Drawing for the job (mm, zero at the part's lowest x, y, z). Round coordinates to 2 decimals unless told otherwise and drop trailing zeros. Loops run counter-clockwise (first coordinate to the right, second up) from the corner with the lowest first, then second, coordinate; pieces in that order, holes last. Notation, with made-up numbers: M 20,28.25 L 64,28.25 A26 cw 64,49.25 Z; hole C -17,57 d10. An arc over 180 degrees is marked long. Use a Markdown table: item, result. Add a question column.
Q1. Cut at C-C (z = 30). Give the cut face in (x, y), plus the area to 3 significant figures.
Q2. Cut at A-A (y = 15). Give the cut face in (x, z).
Q3. Probe line 1 (Y direction, x = 15, z = 29.5); line 2 (X direction, y = 18.5, z = 28.5); line 3 (Y direction, x = 16.5, z = 3.5). List the from-to ranges inside material, lowest first. Write a range as from..to.
Q4. Mould opens along X. For the marked faces 1, 2 and 3 say: +X half, -X half, draft (parallel to the pull), parting line (faces both ways), or undercut.
Q5. Pin check, flat tips, straight feed: pin 1 (1 mm diameter, centred on y = 6.5, z = 31.5, fed in from +X); pin 2 (6 mm diameter, centred on y = 11, z = 16.5, fed in from +X); pin 3 (5 mm diameter, centred on y = 23, z = 31.5, fed in from +X). Stop position of each tip, or through.
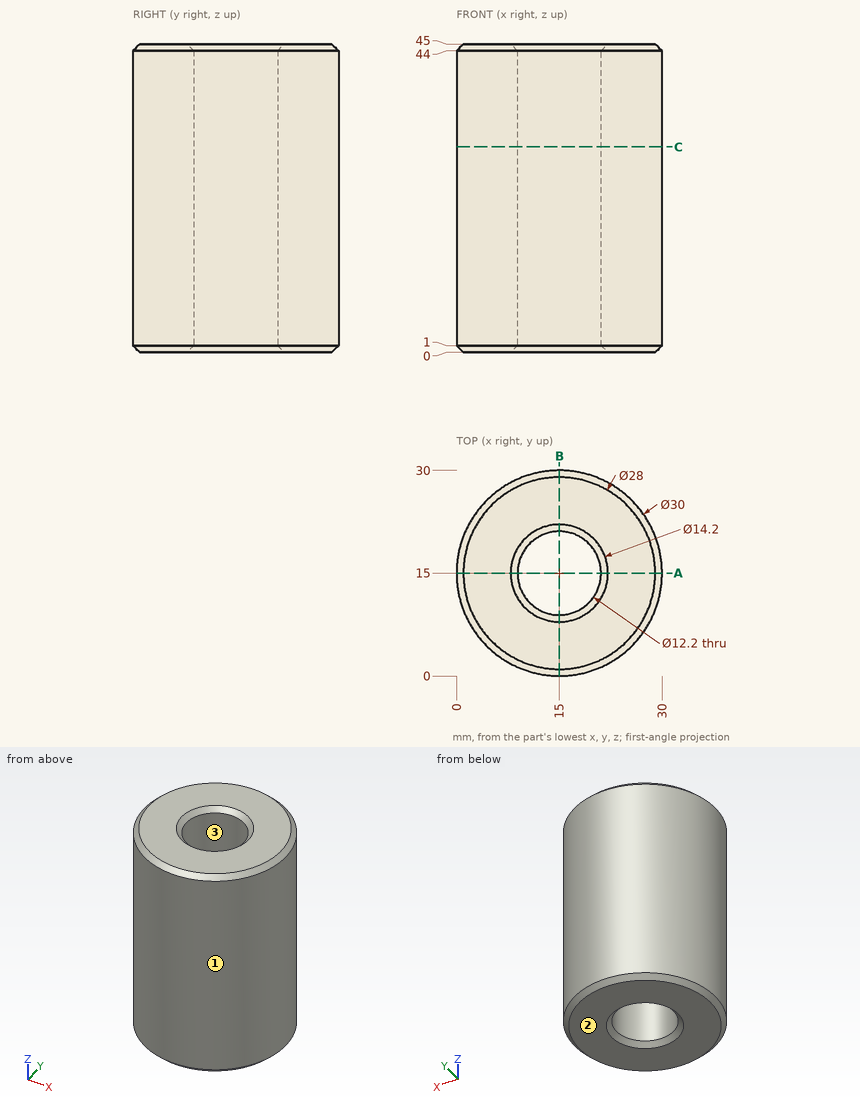
Checked values:
| question | item | result |
|---|---|---|
| 1 | outline | C 15,15 d30; hole C 15,15 d12.2 |
| 1 | area | 590 mm^2 |
| 2 | outline | M 0,1 L 1,0 L 7.9,0 L 8.9,1 L 8.9,44 L 7.9,45 L 1,45 L 0,44 Z; M 21.1,1 L 22.1,0 L 29,0 L 30,1 L 30,44 L 29,45 L 22.1,45 L 21.1,44 Z |
| 3 | line 1 | y = 0..8.9, 21.1..30 |
| 3 | line 2 | x = 0.41..10, 20..29.59 |
| 3 | line 3 | y = 0.08..9.09, 20.91..29.92 |
| 4 | face 1 | parting line |
| 4 | face 2 | draft |
| 4 | face 3 | undercut |
| 5 | pin 1 | stops at x = 27.69 |
| 5 | pin 2 | stops at x = 29.97 |
| 5 | pin 3 | stops at x = 28.96 |
